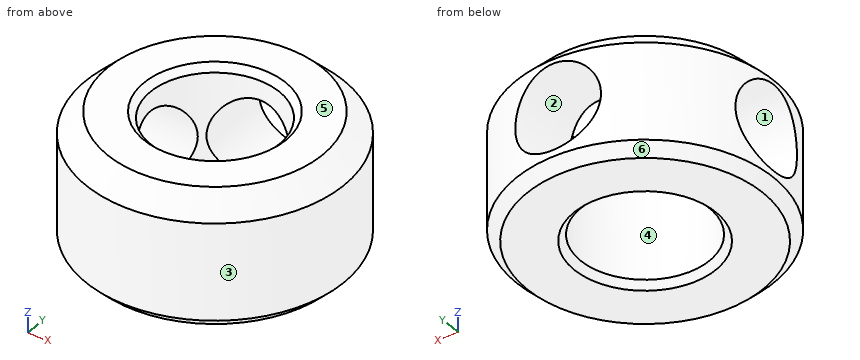
```python
from build123d import *

# Parameters (mm, degrees)
SKETCH_R        = 6
PAD_DEPTH       = 6
SKETCH001_R     = 3
POCKET_DEPTH    = 6.001
CHAMFER_SIZE    = 1
CHAMFER001_SIZE = 0.3
CHAMFER002_SIZE = 0.5
CHAMFER003_SIZE = 0.3
SKETCH002_R     = 2
POCKET001_DEPTH = 6.001
SKETCH003_R     = 2
POCKET002_DEPTH = 6.001


with BuildPart() as part:
    # Sketch → Pad (new body)
    with BuildSketch(Plane.XY):
        Circle(SKETCH_R)
    extrude(amount=PAD_DEPTH)

    # Sketch001 (on Face3 of Pad) → Pocket (cut, through all)
    with BuildSketch(Plane.XY.offset(6)):
        Circle(SKETCH001_R)
    extrude(amount=-POCKET_DEPTH, mode=Mode.SUBTRACT)

    # Chamfer
    chamfer_edges = [part.edges().sort_by_distance(p)[0] for p in [
        (-6, 0, 6),
    ]]
    chamfer(chamfer_edges, length=CHAMFER_SIZE)

    # Chamfer001
    chamfer001_edges = [part.edges().sort_by_distance(p)[0] for p in [
        (-3, 0, 6),
    ]]
    chamfer(chamfer001_edges, length=CHAMFER001_SIZE)

    # Chamfer002
    chamfer002_edges = [part.edges().sort_by_distance(p)[0] for p in [
        (-6, 0, 0),
    ]]
    chamfer(chamfer002_edges, length=CHAMFER002_SIZE)

    # Chamfer003
    chamfer003_edges = [part.edges().sort_by_distance(p)[0] for p in [
        (-3, 0, 0),
    ]]
    chamfer(chamfer003_edges, length=CHAMFER003_SIZE)

    # Sketch002 → Pocket001 (cut, through all)
    with BuildSketch(Plane.YZ):
        with Locations((0, 2.8)):
            Circle(SKETCH002_R)
    extrude(amount=-POCKET001_DEPTH, mode=Mode.SUBTRACT)

    # Sketch003 → Pocket002 (cut, through all)
    with BuildSketch(Plane.XZ):
        with Locations((0, 2.8)):
            Circle(SKETCH003_R)
    extrude(amount=-POCKET002_DEPTH, mode=Mode.SUBTRACT)


solid = part.part
```
Verification items for the finished model (mm, model axes). Face numbers are marked on the shaded views. A direction names the side the tool comes from. Round coordinates to 2 decimals unless told otherwise and drop trailing zeros. Write each loop counter-clockwise with the first axis right and the second up, starting at its lowest first coordinate (ties: lowest second). Pieces come first, ordered by that corner, then holes.
1. Section check A-A on y = 0. Enter the section's corners in (x, z), plus the area to 3 significant figures.
2. Scan lines: L1, parallel to X at y = 0, z = 2.95; L2, parallel to X at y = 3.5, z = 1.65; L3, parallel to Y at x = -4.5, z = 3.4. Record each from-to range of solid material in increasing order.
3. Draft check along X on the marked faces 4, 5 and 6. Enter one of: +X half, -X half, draft (parallel to the pull), parting line (faces both ways), or undercut.
4. Section check C-C on z = 3.05. Enter the section's corners in (x, y).
5. Section check D-D on z = 1.9. Enter the section's corners in (x, y).
6. Section check B-B on x = 0. Enter the section's corners in (y, z).
7. Access from +Z, -Z, +X, -X, +Y, -Y to the whole of each face (thin tool, end or side, straight path). Record for the marked faces 1, 2 and 3.
8. Gauge pin test, flat ends, axial feed: P1, Ø7, axis at x = 0, y = 0, coming from the -Z side; P2, Ø3, axis at x = 4.5, z = 5, coming from the +Y side; P3, Ø1, axis at y = 4.5, z = 4.5, coming from the +X side; P4, Ø3.5, axis at y = 0, z = 2.8, coming from the -X side. Record the tip position at first contact, or that the pin passes through.
Answer:
1. outline: (-6, 0.5) - (-5.5, 0) - (-3.3, 0) - (-3, 0.3) - (-3, 0.8) - (-6, 0.8) - close; (-6, 4.8) - (-3, 4.8) - (-3, 5.7) - (-3.3, 6) - (-5, 6) - (-6, 5) - close; (3, 0.3) - (3.3, 0) - (5.5, 0) - (6, 0.5) - (6, 5) - (5, 6) - (3.3, 6) - (3, 5.7) - close
1. area: 22.6 mm2
2. L1: x = 3 to 6
2. L2: x = -4.87 to -1.64, 1.64 to 4.87
2. L3: y = -3.97 to -1.91, 1.91 to 3.97
3. face 4: undercut
3. face 5: draft
3. face 6: parting line
4. outline: (-5.66, -1.98) arc R6 ccw (long way) to (1.98, 5.66) - (1.98, 2.25) arc R3 cw (long way) to (-2.25, -1.98) - close; (-5.66, 1.98) - (-2.25, 1.98) arc R3 cw to (-1.98, 2.25) - (-1.98, 5.66) arc R6 ccw to start
5. outline: (-5.73, -1.79) arc R6 ccw (long way) to (1.79, 5.73) - (1.79, 2.41) arc R3 cw (long way) to (-2.41, -1.79) - close; (-5.73, 1.79) - (-2.41, 1.79) arc R3 cw to (-1.79, 2.41) - (-1.79, 5.73) arc R6 ccw to start
6. outline: (-6, 0.5) - (-5.5, 0) - (-3.3, 0) - (-3, 0.3) - (-3, 5.7) - (-3.3, 6) - (-5, 6) - (-6, 5) - close; (3, 0.3) - (3.3, 0) - (5.5, 0) - (6, 0.5) - (6, 0.8) - (3, 0.8) - close; (3, 4.8) - (6, 4.8) - (6, 5) - (5, 6) - (3.3, 6) - (3, 5.7) - close
7. face 1: -X
7. face 2: +Y
7. face 3: +Z, -Z
8. P1: stops at z = 0
8. P2: stops at y = 5.2
8. P3: stops at x = 4.47
8. P4: stops at x = 2.44
